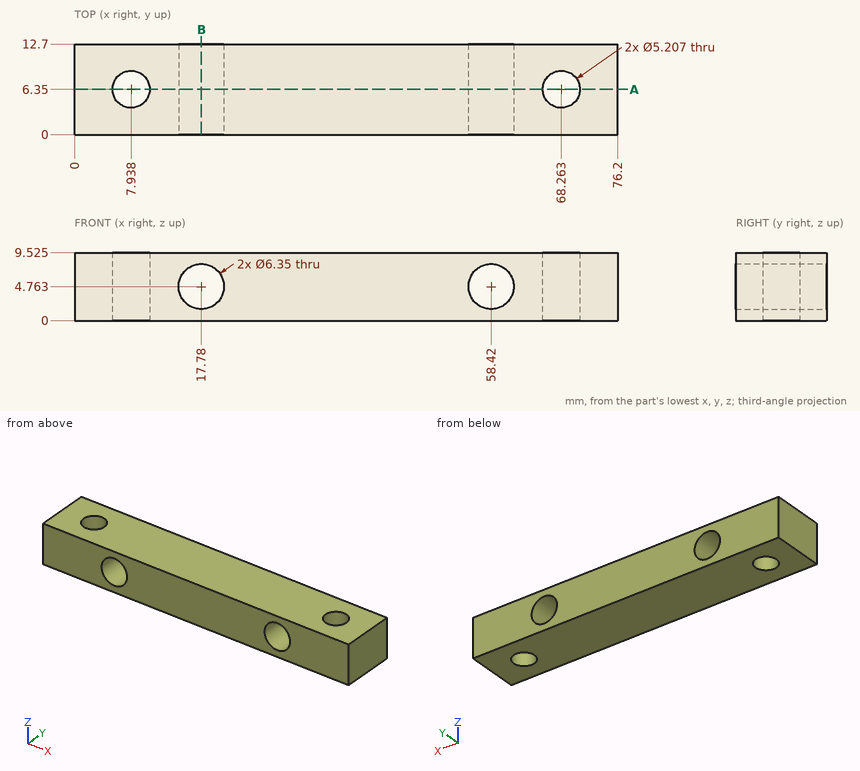
Here's the drawing with two shaded views (mm, measured from the low corner). I have some questions. Coordinates: 2 decimals unless noted, no trailing zeros. Loops run counter-clockwise (first coordinate to the right, second up) from the corner with the lowest first, then second, coordinate; pieces in that order, holes last. Notation, with made-up numbers: (63.5, 2) - (119.5, 2) arc R19 cw to (119.5, 6) - close; hole circle Ø2 at (18.25, 38.25). An arc over 180 degrees is marked (long way). Answer as CSV lines item,"result". Start each with the question number.
1) Suppose I cut it at A-A (y = 6.35). Count the separate pieces of the cut face and the enclosed holes in it.
2) Suppose I cut it at B-B (x = 17.78). Please give me the cut outline in (y, z) (1 decimal).
3) I need wall thicknesses on line 1 (X direction, y = 10.25, z = 5) (1 decimal); line 2 (X direction, y = 9.25, z = 3.25); line 3 (X direction, y = 4.25, z = 5.75) (1 decimal). Which ranges of each line are inside material? Lowest first, please. Write a range as from..to.
Check result:
1,separate pieces,"3"
1,enclosed holes,"2"
2,outline,"(0, 0) - (12.7, 0) - (12.7, 1.6) - (0, 1.6) - close; (0, 7.9) - (12.7, 7.9) - (12.7, 9.5) - (0, 9.5) - close"
3,line 1,"x = 0..14.6, 20.9..55.3, 61.6..76.2"
3,line 2,"x = 0..14.99, 20.57..55.63, 61.21..76.2"
3,line 3,"x = 0..6.4, 9.5..14.8, 20.8..55.4, 61.4..66.7, 69.8..76.2"
